Source: CAD feature listing. Evaluate the final solid. Frame: model axes, mm. A direction names the side the tool comes from. Give positions to 0.01 mm unless a question says otherwise; leave off trailing zeros. Order: outer loops, then holes, each group sorted by start corner. A loop starts at its lowest first (then second) coordinate and runs counter-clockwise, first axis right, second up.
from build123d import *

# Parameters (mm, degrees)
F0_W     = 238.125
F0_H     = 168.275
F1_DEPTH = 6.35
F3_DEPTH = 25.4
F4_R     = 5.08
F5_DEPTH = 6.351
F7_DEPTH = 6.351


with BuildPart() as f1:
    # F0 (on Top) → F1 (new body)
    with BuildSketch(Plane.XY):
        Rectangle(F0_W, F0_H)
    extrude(amount=F1_DEPTH)

    # F2 (on face) → F3 (cut)
    with BuildSketch(Plane.XY.offset(6.35)):
        Polygon((23.3045, 43.8785), (-66.6115, -46.0375), (68.2625, -46.0375), (68.2625, 43.8785), align=None)
    extrude(amount=-F3_DEPTH, mode=Mode.SUBTRACT)

    # F4
    f4_edges = [f1.edges().sort_by_distance(p)[0] for p in [
        (119.0625, -84.1375, 3.175),
        (119.0625, 84.1375, 3.175),
        (-119.0625, -84.1375, 3.175),
        (-119.0625, 84.1375, 3.175),
    ]]
    fillet(f4_edges, radius=F4_R)

    # F2 (on face) → F5 (cut, through all)
    with BuildSketch(Plane.XY.offset(6.35)):
        Polygon((23.3045, 43.8785), (-66.6115, -46.0375), (68.2625, -46.0375), (68.2625, 43.8785), align=None)
    extrude(amount=-F5_DEPTH, mode=Mode.SUBTRACT)

    # F6 (on face) → F7 (cut, through all)
    with BuildSketch(Plane.XY.offset(6.35)):
        with BuildLine():
            Line((68.7451, 45.1485), (23.104601, 45.1485))
            ThreePointArc((23.104601, 45.1485), (22.803276, 45.088563), (22.547825, 44.917876))
            Line((22.547825, 44.917876), (-68.333375, -45.963324))
            ThreePointArc((-68.333375, -45.963324), (-68.504062, -46.821425), (-67.776599, -47.3075))
            Line((-67.776599, -47.3075), (68.7451, -47.3075))
            ThreePointArc((68.7451, -47.3075), (69.301876, -47.076876), (69.5325, -46.5201))
            Line((69.5325, -46.5201), (69.5325, 44.3611))
            ThreePointArc((69.5325, 44.3611), (69.301876, 44.917876), (68.7451, 45.1485))
        make_face()
    extrude(amount=-F7_DEPTH, mode=Mode.SUBTRACT)


solid = f1.part
(1) Line query: line 1 along Y through (x, z) = (29, 2.5); line 2 along X through (y, z) = (31, 1.75); line 3 along X through (y, z) = (24.5, 4.5). Output: solid intervals per line, ascending.
(2) Draft query along X for faces 1 (the flat face through (46, 45.148, 3)), 2 (the flat face through (-2, 84.138, 3)), 3 (the flat face through (-119.062, -1, 3)). Return one class per face: +X half, -X half, draft (parallel to the pull), parting line (faces both ways), or undercut.
(3) Section C-C, the plane y = -15. Return loops of the section in (x, z).
(4) Section B-B, the plane z = 1.75. Return loops of the section in (x, y), plus the area to 3 significant figures.
(5) Access query for faces 4 (the flat face through (119.062, -1, 3)), 5 (the flat face through (69.532, -2, 3)). Directions: +Z, -Z, +X, -X, +Y, -Y. A direction counts if a zero-diameter tool reaches every point of the face in a straight line with its end or side. Return the directions, or none.
(6) Section A-A, the plane x = 66. Return loops of the section in (y, z).
Checks:
1. line 1: y = -84.14 to -47.31, 45.15 to 84.14
1. line 2: x = -119.06 to 8.63, 69.53 to 119.06
1. line 3: x = -119.06 to 2.13, 69.53 to 119.06
2. face 1: undercut
2. face 2: draft
2. face 3: -X half
3. outline: (-119.06, 0) - (-37.37, 0) - (-37.37, 6.35) - (-119.06, 6.35) - close; (69.53, 0) - (119.06, 0) - (119.06, 6.35) - (69.53, 6.35) - close
4. outline: (-119.06, -79.06) arc R5.08 ccw to (-113.98, -84.14) - (113.98, -84.14) arc R5.08 ccw to (119.06, -79.06) - (119.06, 79.06) arc R5.08 ccw to (113.98, 84.14) - (-113.98, 84.14) arc R5.08 ccw to (-119.06, 79.06) - close; hole (-68.33, -45.96) arc R0.79 ccw to (-67.78, -47.31) - (68.75, -47.31) arc R0.79 ccw to (69.53, -46.52) - (69.53, 44.36) arc R0.79 ccw to (68.75, 45.15) - (23.1, 45.15) arc R0.79 ccw to (22.55, 44.92) - close
4. area: 31,500 mm2
5. face 4: +Z, -Z, +X, +Y, -Y
5. face 5: +Z, -Z
6. outline: (-84.14, 0) - (-47.31, 0) - (-47.31, 6.35) - (-84.14, 6.35) - close; (45.15, 0) - (84.14, 0) - (84.14, 6.35) - (45.15, 6.35) - close
